Source: CAD feature listing. Evaluate the final solid. Frame: model axes, mm. Coordinates: 2 decimals unless noted, no trailing zeros. Loops run counter-clockwise (first coordinate to the right, second up) from the corner with the lowest first, then second, coordinate; pieces in that order, holes last. Notation, with made-up numbers: (32, 57.25) -> (77, 57.25) arc R19 cw to (77, 85.25) -> close; hole circle Ø8 at (14, 47). An arc over 180 degrees is marked (long way). One line per question, with ' | ' between items. Start each with the question number.
Autodesk Inventor part; units mm, degrees
ref_plane "YZ Plane" through (0, 0, 0) normal (1, 0, 0) x (0, 1, 0)
ref_plane "XZ Plane" through (0, 0, 0) normal (0, 1, 0) x (-1, 0, 0)
ref_plane "XY Plane" through (0, 0, 0) normal (0, 0, 1) x (1, 0, 0)
sketch "Sketch1" plane through (0, 0, 0) normal (0, 1, 0) x (-1, 0, 0)
  circle A0 centre (0, 0) radius 3.175
  circle A1 centre (95.25, 0) radius 3.175
  line L0 (95.25, 6.35) -> (0, 6.35)
  line L1 (95.25, -6.35) -> (0, -6.35)
  line L2 (95.25, 0) -> (0, 0) construction
  arc A2 (95.25, -6.35) -> (95.25, 6.35) centre (95.25, 0) ccw
  arc A3 (0, 6.35) -> (0, -6.35) centre (0, 0) ccw
  circle A4 centre (47.625, 0) radius 3.175
  dimension "d0" = 6.35
  dimension "d1" = 6.35
  dimension "d2" = 95.25
  dimension "d3" = 12.7
  dimension "d4" = 6.35
extrude "Extrusion1" add sketch "Sketch1" along normal blind 3.175
sketch "Sketch2" plane through (0, 3.175, 0) normal (0, 1, 0) x (1, 0, 0)
  circle A0 centre (0, 0) radius 6.35
  circle A1 centre (0, 0) radius 31.75
  dimension "d7" = 12.7
  dimension "d8" = 63.5
extrude "Extrusion2" [suppressed]
sketch "Sketch3" plane through (0, 3.175, 0) normal (0, 1, 0) x (1, 0, 0)
  line L0 (-3.6662, 6.35) -> (3.6662, 6.35)
  line L1 (3.6662, 6.35) -> (7.3323, 0)
  line L2 (7.3323, 0) -> (3.6662, -6.35)
  line L3 (3.6662, -6.35) -> (-3.6662, -6.35)
  line L4 (-3.6662, -6.35) -> (-7.3323, 0)
  line L5 (-7.3323, 0) -> (-3.6662, 6.35)
  circle A0 centre (-23.8125, 0) radius 2.54
  circle A1 centre (0, 0) radius 23.8125 construction
  circle A2 centre (-11.9062, -20.6222) radius 2.54
  circle A3 centre (11.9062, -20.6222) radius 2.54
  circle A4 centre (23.8125, 0) radius 2.54
  circle A5 centre (11.9062, 20.6222) radius 2.54
  circle A6 centre (-11.9063, 20.6222) radius 2.54
  circle A7 centre (0, 0) radius 12.7
  arc A8 (-31.1085, -6.35) -> (-31.1085, 6.35) centre (0, 0) ccw
  line L6 (-31.1085, -6.35) -> (-2.6494, -12.4206)
  line L7 (0, 6.35) -> (-95.25, 6.35)
  line L8 (-31.1085, 6.35) -> (-2.6494, 12.4206)
  dimension "d13" = 47.625
  dimension "d11" = 12.7
  dimension "d12" = 5.08
  dimension "d16" = 360
  dimension "d20" = 25.4
extrude "Extrusion3" [suppressed]
properties part number "OUTK_019_PanikSiscior" material "Aluminum 6061"
(1) Draft query along X for faces 1 (the cylindrical face through (6.35, 1.57, -0.14)), 2 (the cylindrical face through (-101.6, 1.6, 0.1)), 3 (the cylindrical face through (0.69, 1.57, 3.1)), 4 (the flat face through (-47, 3.175, 4)). Return one class per face: pulls with the +X half, pulls with the -X half, needs draft (parallel to the pull), parting line crosses it, or undercut.
(2) Contact query for a flat-ended pin moving along its axis: pin 1 Ø4 at (x, z) = (-47.625, 0) entering from +Y. Output: stop coordinate, or through.
(3) Cut plane B-B, the plane y = 0.9. Return the cut outline in (x, z) (3 decimals).
(4) Cut plane A-A, the plane z = 0. Return the cut outline in (x, y) (3 decimals), and give its area (3 significant figures).
(5) Ray query, L1, parallel to Z at x = 0, y = 2.15 (3 decimals); L2, parallel to X at y = 0.85, z = 2.5; L3, parallel to X at y = 2.4, z = 1.25. Return the intervals inside material, ascending.
Here are the results:
1) face 1: pulls with the +X half | face 2: pulls with the -X half | face 3: undercut | face 4: needs draft
2) pin 1: passes through
3) outline: (-95.25, -6.35) -> (0, -6.35) arc R6.35 ccw to (0, 6.35) -> (-95.25, 6.35) arc R6.35 ccw to start; hole circle Ø6.35 at (-95.25, 0); hole circle Ø6.35 at (-47.625, 0); hole circle Ø6.35 at (0, 0)
4) outline: (-101.6, 0) -> (-98.425, 0) -> (-98.425, 3.175) -> (-101.6, 3.175) -> close; (-92.075, 0) -> (-50.8, 0) -> (-50.8, 3.175) -> (-92.075, 3.175) -> close; (-44.45, 0) -> (-3.175, 0) -> (-3.175, 3.175) -> (-44.45, 3.175) -> close; (3.175, 0) -> (6.35, 0) -> (6.35, 3.175) -> (3.175, 3.175) -> close | area: 282 mm2
5) L1: z = -6.35 to -3.175, 3.175 to 6.35 | L2: x = -101.09 to -97.21, -93.29 to -49.58, -45.67 to -1.96, 1.96 to 5.84 | L3: x = -101.48 to -98.17, -92.33 to -50.54, -44.71 to -2.92, 2.92 to 6.23
